Autodesk Inventor part; units mm, degrees
ref_plane "YZ Plane" through (0, 0, 0) normal (1, 0, 0) x (0, 1, 0)
ref_plane "XZ Plane" through (0, 0, 0) normal (0, 1, 0) x (-1, 0, 0)
ref_plane "XY Plane" through (0, 0, 0) normal (0, 0, 1) x (1, 0, 0)
sketch "Sketch1" plane through (0, 0, 0) normal (0, 1, 0) x (-1, 0, 0)
  circle A0 centre (0, 0) radius 17
  dimension "d0" = 34
extrude "Extrusion1" add sketch "Sketch1" along normal blind 2
sketch "Sketch2" plane through (0, 0, 0) normal (0, -1, 0) x (1, 0, 0)
  circle A0 centre (0, 0) radius 17
  circle A1 centre (0, 0) radius 15
  dimension "d3" = 2
extrude "Extrusion2" add sketch "Sketch2" along normal blind 1
sketch "Sketch3" plane through (0, 2, 0) normal (0, 1, 0) x (1, 0, 0)
  circle A0 centre (0, 0) radius 17
  arc A1 (-9.1924, -9.1924) -> (9.1924, -9.1924) centre (0, 0) ccw
  arc A2 (-7.7782, -7.7782) -> (7.7782, -7.7782) centre (0, 0) ccw
  line L0 (0, 0) -> (-9.1924, -9.1924) construction
  line L1 (0, 0) -> (9.1924, -9.1924) construction
  line L2 (-9.1924, -9.1924) -> (-7.7782, -7.7782)
  line L3 (7.7782, -7.7782) -> (9.1924, -9.1924)
  dimension "d6" = 4
  dimension "d7" = 2
extrude "Extrusion3" cut sketch "Sketch3" against normal through all contours L2 A2 L3 A1
mirror "Mirror1" about plane through (0, 0, 0) normal (0, 0, 1) of "Extrusion3"
properties part number "circularholder" material "PET Plastic"
The listing builds one solid part. Answer for the finished solid, in the listing's coordinates (mm). A direction names the side the tool comes from. Coordinates: 2 decimals unless noted, no trailing zeros. Write each loop counter-clockwise with the first axis right and the second up, starting at its lowest first coordinate (ties: lowest second). Pieces come first, ordered by that corner, then holes. Notation, with made-up numbers: (-35, 51.25) - (4, 51.25) arc R13 cw to (4, 75.25) - close; hole circle Ø1 at (83, 66). An arc over 180 degrees is marked (long way). Return JSON: item names as keys, results as strings. Group by question number.
1. A cutting plane is placed at D-D, the plane z = 0. Determine the outline of the cut face in (x, y).
2. A cutting plane is placed at C-C, the plane y = 1.05. Determine the outline of the cut face in (x, z).
3. Given pin 1 (2 mm diameter, centred on x = 5.5, z = 1.5, fed in from -Y), flat-ended and moving along its own axis, determine where the tip first touches the part or whether it passes through.
4. A cutting plane is placed at B-B, the plane z = -8.5. Determine the outline of the cut face in (x, y), plus the area to 3 significant figures.
5. A cutting plane is placed at A-A, the plane x = 0. Determine the outline of the cut face in (y, z).
6. Which of the six approach directions +Z, -Z, +X, -X, +Y, -Y give full straight-line access (tool end or side, diameter ignored) to faces 1 (the flat face through (8, 1, -8)), 2 (the cylindrical face through (-14.985, -0.493, -0.66)), 3 (the flat face through (0, 2, 0))?
7. Straight lines are drawn through the part: L1, parallel to Z at x = 0, y = -0.2; L2, parallel to Z at x = 0.5, y = 1; L3, parallel to Y at x = -8.5, z = -1.5. For each, find the intervals that lie inside material, in ascending order.
8. Determine the mould class of faces 4 (the flat face through (0, 0, 0)), 5 (the flat face through (6, -1, -14)) for opening direction X: released by +X, released by -X, zero draft, split by the parting line, or undercut.
Ans:
{
 "1": {"outline": "(-17, -1) - (-15, -1) - (-15, 0) - (15, 0) - (15, -1) - (17, -1) - (17, 2) - (-17, 2) - close"},
 "2": {"outline": "circle Ø34 at (0, 0); hole (-9.19, -9.19) arc R13 ccw to (9.19, -9.19) - (7.78, -7.78) arc R11 cw to (-7.78, -7.78) - close; hole (-9.19, 9.19) - (-7.78, 7.78) arc R11 cw to (7.78, 7.78) - (9.19, 9.19) arc R13 ccw to start"},
 "3": {"pin 1": "y = 0"},
 "4": {"outline": "(-14.72, -1) - (-12.36, -1) - (-12.36, 0) - (-8.5, 0) - (-8.5, 2) - (-14.72, 2) - close; (-6.98, 0) - (6.98, 0) - (6.98, 2) - (-6.98, 2) - close; (8.5, 0) - (12.36, 0) - (12.36, -1) - (14.72, -1) - (14.72, 2) - (8.5, 2) - close", "area": "57.5 mm²"},
 "5": {"outline": "(-1, -17) - (2, -17) - (2, -13) - (0, -13) - (0, -15) - (-1, -15) - close; (-1, 15) - (0, 15) - (0, 13) - (2, 13) - (2, 17) - (-1, 17) - close; (0, -11) - (2, -11) - (2, 11) - (0, 11) - close"},
 "6": {"face 1": "+Y, -Y", "face 2": "-Y", "face 3": "+Z, -Z, +X, -X, +Y"},
 "7": {"L1": "-17 to -15, 15 to 17", "L2": "-16.99 to -12.99, -10.99 to 10.99, 12.99 to 16.99", "L3": "0 to 2"},
 "8": {"face 4": "undercut", "face 5": "zero draft"}
}
